Check sheet for the modelled part. Datum: model origin and axes. Units: mm. A direction names the side the tool comes from. Give positions to 0.01 mm unless a question says otherwise; leave off trailing zeros. Loops run counter-clockwise (first coordinate to the right, second up) from the corner with the lowest first, then second, coordinate; pieces in that order, holes last.
```python
from build123d import *

# Parameters (mm, degrees)
SKETCH1_W           = 34
SKETCH1_H           = 18.5
BOSS_EXTRUDE1_DEPTH = 2
SKETCH2_W           = 4
SKETCH2_H           = 6
BOSS_EXTRUDE2_DEPTH = 1
SKETCH3_W           = 2
SKETCH3_H           = 4
BOSS_EXTRUDE3_DEPTH = 1
BOSS_EXTRUDE4_DEPTH = 1


with BuildPart() as part:
    # Sketch1 → Boss-Extrude1 (new body)
    with BuildSketch(Plane(origin=(0, 0, 0), x_dir=(1, 0, 0), z_dir=(0, 1, 0))):
        Rectangle(SKETCH1_W, SKETCH1_H)
    extrude(amount=BOSS_EXTRUDE1_DEPTH)

    # Sketch2 → Boss-Extrude2 (add)
    with BuildSketch(Plane(origin=(0, 2, 0), x_dir=(1, 0, 0), z_dir=(0, 1, 0))):
        with Locations((11.5, 0)):
            Rectangle(SKETCH2_W, SKETCH2_H)
    extrude(amount=BOSS_EXTRUDE2_DEPTH)

    # Sketch3 → Boss-Extrude3 (add)
    with BuildSketch(Plane(origin=(0, 3, 0), x_dir=(1, 0, 0), z_dir=(0, 1, 0))):
        with Locations((11.5, 0)):
            Rectangle(SKETCH3_W, SKETCH3_H)
    extrude(amount=BOSS_EXTRUDE3_DEPTH)

    # Sketch4 → Boss-Extrude4 (add)
    with BuildSketch(Plane(origin=(0, 2, 0), x_dir=(1, 0, 0), z_dir=(0, 1, 0))):
        Polygon((3.5, 0), (-1.449747468, 4.949747468), (-6.399494937, 0), (-1.449747468, -4.949747468), align=None)
    extrude(amount=BOSS_EXTRUDE4_DEPTH)


solid = part.part
```
(1) Gauge pin test, flat ends, axial feed: pin 1 Ø0.8 at (x, y) = (11.5, 2.5) entering from +Z; pin 2 Ø2 at (x, y) = (0, 2.5) entering from -Z; pin 3 Ø0.8 at (x, y) = (12, 2.5) entering from -Z; pin 4 Ø0.5 at (y, z) = (3.5, 0) entering from -X. Record the tip position at first contact, or that the pin passes through.
(2) Release check for a two-part mould opening along X. For faces 1 (the face through (1.1, 2.5, -2.4)), 2 (the face through (13.5, 2.5, 0)), 3 (the face through (-3.9, 2.5, -2.5)) record: pulls with the +X half, pulls with the -X half, needs draft (parallel to the pull), parting line crosses it, or undercut.
(3) Section check C-C on x = -3.5. Record the boundary of the cut face in (y, z), plus the area to 3 significant figures.
(4) Section check A-A on y = 2.5. Record the boundary of the cut face in (x, z), plus the area to 3 significant figures.
(5) Access from +Z, -Z, +X, -X, +Y, -Y to the whole of each face (thin tool, end or side, straight path). Record for faces 4 (the face through (1, 2.5, 2.5)), 5 (the face through (12.5, 3.5, 0)), 6 (the face through (-2, 3, 0)), 7 (the face through (11.5, 3.5, 2)).
(6) Section check B-B on z = -0.75. Record the boundary of the cut face in (x, y), plus the area to 3 significant figures.
(7) Section check D-D on z = -4.5. Record the boundary of the cut face in (x, y).
(8) Material ranges on line 1 (Y direction, x = -13.5, z = 4.5); line 2 (X direction, y = 2.7, z = -1.5); line 3 (X direction, y = 2.55, z = -0.5), recorded low to high.
Computed values:
1. pin 1: stops at z = 3
1. pin 2: stops at z = -9.25
1. pin 3: stops at z = -3
1. pin 4: stops at x = 10.5
2. face 1: undercut
2. face 2: pulls with the +X half
2. face 3: pulls with the -X half
3. outline: (0, -9.25) - (2, -9.25) - (2, -2.9) - (3, -2.9) - (3, 2.9) - (2, 2.9) - (2, 9.25) - (0, 9.25) - close
3. area: 42.8 mm2
4. outline: (-6.4, 0) - (-1.45, -4.95) - (3.5, 0) - (-1.45, 4.95) - close; (9.5, -3) - (13.5, -3) - (13.5, 3) - (9.5, 3) - close
4. area: 73.0 mm2
5. face 4: +Z, +Y
5. face 5: +Z, -Z, +X, +Y
5. face 6: +Z, -Z, -X, +Y
5. face 7: +Z, +X, -X, +Y
6. outline: (-17, 0) - (17, 0) - (17, 2) - (13.5, 2) - (13.5, 3) - (12.5, 3) - (12.5, 4) - (10.5, 4) - (10.5, 3) - (9.5, 3) - (9.5, 2) - (2.75, 2) - (2.75, 3) - (-5.65, 3) - (-5.65, 2) - (-17, 2) - close
6. area: 82.4 mm2
7. outline: (-17, 0) - (17, 0) - (17, 2) - (-1, 2) - (-1, 3) - (-1.9, 3) - (-1.9, 2) - (-17, 2) - close
8. line 1: y = 0 to 2
8. line 2: x = -4.9 to 2, 9.5 to 13.5
8. line 3: x = -5.9 to 3, 9.5 to 13.5
